Job drawing, mm, ordinate dimensions from the low corner. One solid piece. A direction names the side the tool comes from. Give positions to 0.01 mm unless a question says otherwise; leave off trailing zeros. Order: outer loops, then holes, each group sorted by start corner. A loop starts at its lowest first (then second) coordinate and runs counter-clockwise, first axis right, second up. Notation, with made-up numbers: (41.25, 86.25) - (66.25, 86.25) arc R38 cw to (66.25, 124.25) - close; hole circle Ø5 at (-23, -20). An arc over 180 degrees is marked (long way). Use one line per item in the form item = value. Start each with the question number.
1. Drill centre lines: line 1 (Y direction, x = 37, z = 1); line 2 (X direction, y = 19.5, z = 24); line 3 (Y direction, x = 7.5, z = 6). Where is each one in solid material? Low to high.
2. Pull direction Y, two halves, no side cores. Call the marked faces 4, 5 and 6: +Y half, -Y half, draft (parallel to the pull), parting line (faces both ways), or undercut.
3. Band-saw the part on A-A, the plane z = 17.78. List the corners of the cut face in (x, y), plus the area to 3 significant figures.
4. Band-saw the part on B-B, the plane x = 39. List the corners of the cut face in (y, z).
5. Tool access for the marked faces 1, 2 and 3: list every direction of +Z, -Z, +X, -X, +Y, -Y with a clear straight run to the whole face (end or side of a thin tool).
6. Band-saw the part on D-D, the plane z = 22.5. List the corners of the cut face in (x, y).
7. Band-saw the part on C-C, the plane y = 15. List the corners of the cut face in (x, z), plus the area to 3 significant figures.
8. Pin check, flat tips, straight feed: P1, Ø1.4, axis at y = 44.5, z = 26.5, coming from the -X side; P2, Ø4, axis at x = 27, z = 19, coming from the -Y side; P3, Ø8, axis at x = 16.5, z = 20, coming from the +Y side. Stop position of each tip, or through.
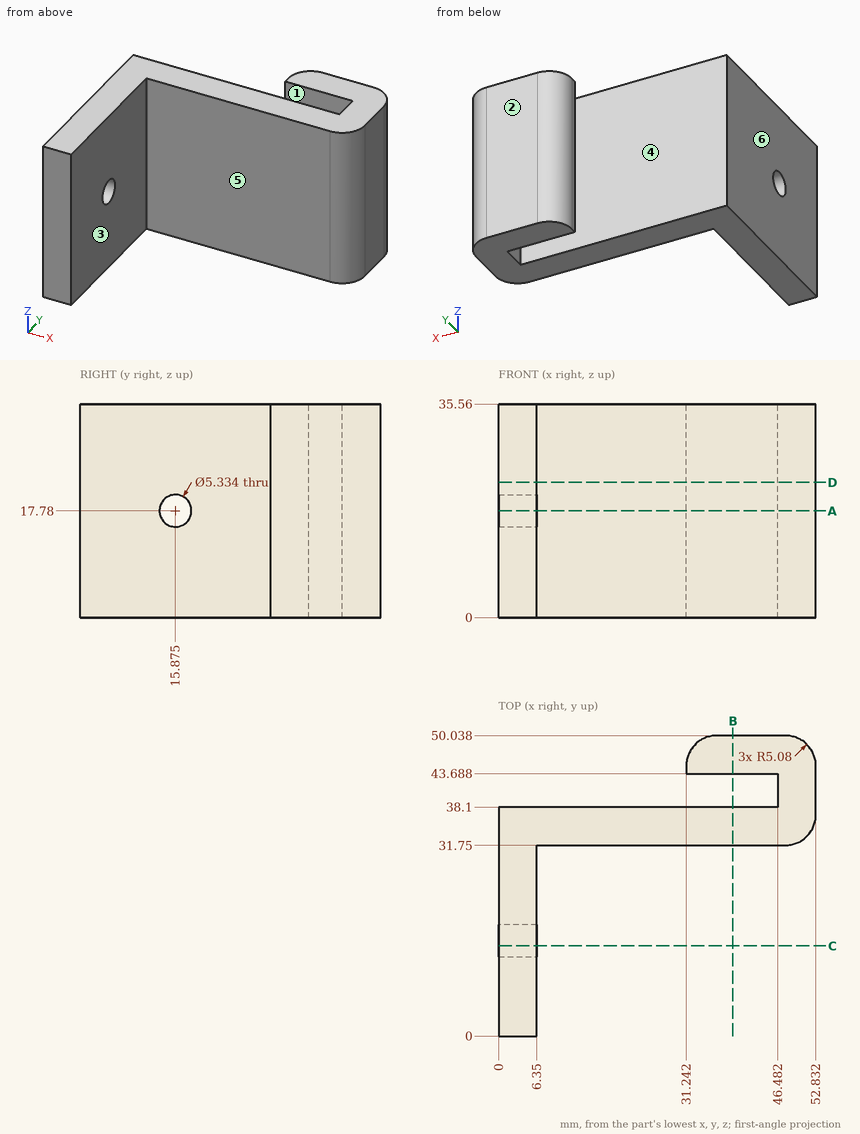
From the geometry:
q1.line_1 = 31.75 to 38.1, 43.69 to 50.04
q1.line_2 = 0 to 6.35
q1.line_3 = 31.75 to 38.1
q2.face_4 = undercut
q2.face_5 = -Y half
q2.face_6 = draft
q3.outline = (0, 0) - (6.35, 0) - (6.35, 13.21) - (0, 13.21) - close; (0, 18.54) - (6.35, 18.54) - (6.35, 31.75) - (47.75, 31.75) arc R5.08 ccw to (52.83, 36.83) - (52.83, 44.96) arc R5.08 ccw to (47.75, 50.04) - (36.32, 50.04) arc R5.08 ccw to (31.24, 44.96) - (31.24, 43.69) - (46.48, 43.69) - (46.48, 38.1) - (0, 38.1) - close
q3.area = 659 mm²
q4.outline = (31.75, 0) - (38.1, 0) - (38.1, 35.56) - (31.75, 35.56) - close; (43.69, 0) - (50.04, 0) - (50.04, 35.56) - (43.69, 35.56) - close
q5.face_1 = +Z, -Z, -X
q5.face_2 = +Z, -Z, +X, -X, +Y
q5.face_3 = +Z, -Z, +X, -Y
q6.outline = (0, 0) - (6.35, 0) - (6.35, 31.75) - (47.75, 31.75) arc R5.08 ccw to (52.83, 36.83) - (52.83, 44.96) arc R5.08 ccw to (47.75, 50.04) - (36.32, 50.04) arc R5.08 ccw to (31.24, 44.96) - (31.24, 43.69) - (46.48, 43.69) - (46.48, 38.1) - (0, 38.1) - close
q7.outline = (0, 0) - (6.35, 0) - (6.35, 15.26) - (0, 15.26) - close; (0, 20.3) - (6.35, 20.3) - (6.35, 35.56) - (0, 35.56) - close
q7.area = 194 mm²
q8.P1 = 31.24
q8.P2 = 31.75
q8.P3 = 38.1
